For this review, take the finished solid that the model builds, in its own axes (mm). A direction names the side the tool comes from. Round coordinates to 2 decimals unless told otherwise and drop trailing zeros. Write each loop counter-clockwise with the first axis right and the second up, starting at its lowest first coordinate (ties: lowest second). Pieces come first, ordered by that corner, then holes. Notation, with made-up numbers: (47.5, -40) -> (94.5, -40) arc R31 cw to (94.5, -1) -> close; hole circle Ø8 at (14, -32.5). An arc over 180 degrees is marked (long way). Answer as CSV lines item,"result". Start each with the question number.
Item 1: Take a section at B-B on z = -17.75. Count the separate pieces of the cut face and the enclosed holes in it, then the cut area to 3 significant figures.
Item 2: Machinability: for faces 4 (the cylindrical face through (-28.95, -54.45, -25.09)), 5 (the cylindrical face through (5.325, 32.732, -13.727)), 6 (the flat face through (-7.605, -12.93, -4.93)), which of the approach directions +Z, -Z, +X, -X, +Y, -Y give a long, thin tool a straight path to every point of the face, cutting with its end or side? Answer none if there is none.
Item 3: Wall thickness on probe 1 along X at (y, z) = (-24, -4.5); probe 2 along X at (y, z) = (-38, -24.25); probe 3 along Y at (x, z) = (-32.5, -24.25): over which ranges is each line inside the solid? List them lowest first. Write a range as from..to.
Item 4: For pin 1 Ø8 at (y, z) = (14, -23) entering from -X; pin 2 Ø5.5 at (x, y) = (-65, 0) entering from -Z (3 decimals); pin 3 Ø5 at (y, z) = (-54.5, -9.5) entering from +X, all flat-tipped, find the tip position at first contact; note any pin that passes through.
Item 5: Mouldability with a two-part tool opening along X and no side actions: class faces 1 (the flat face through (15, 0, -5)), 2 (the flat face through (16, 1, 0)), 3 (the cylindrical face through (-9.764, 74.362, -13.348)) as +X half, -X half, draft (parallel to the pull), parting line (faces both ways), or undercut.
Item 6: Take a section at A-A on x = 65. Give the boundary of the cut face in (y, z) (3 decimals), then the cut area to 3 significant figures.
```python
from build123d import *

# Parameters (mm, degrees)
ESBO_O1_R                        = 75
RESSALTO_EXTRUS_O1_DEPTH         = 27.075013067
ESBO_O2_R                        = 8.8
CORTE_EXTRUS_O1_DEPTH            = 110.467147275
CORTE_EXTRUS_O2_DEPTH            = 10
REBAIXO_PARA_SHCS_M41_AT_2_COUNT = 2
REBAIXO_PARA_SHCS_M41_AT_2_PITCH = 65
REBAIXO_PARA_SHCS_M41_AT_3_COUNT = 2
REBAIXO_PARA_SHCS_M41_AT_3_PITCH = 112.583302492
REBAIXO_PARA_SHCS_M41_AT_4_COUNT = 2
REBAIXO_PARA_SHCS_M41_AT_4_PITCH = 130
REBAIXO_PARA_SHCS_M41_AT_5_COUNT = 2
REBAIXO_PARA_SHCS_M41_AT_5_PITCH = 65
REBAIXO_PARA_SHCS_M41_AT_6_COUNT = 2
REBAIXO_PARA_SHCS_M41_AT_6_PITCH = 112.583302492
CORTE_EXTRUS_O3_DEPTH            = 110.467147275
PADR_OCIRCULAR1_COUNT            = 5
ESBO_O9_R                        = 4


with BuildPart() as part:
    # Esboço1 → Ressalto-extrusão1 (new body)
    with BuildSketch(Plane.XY):
        Circle(ESBO_O1_R)
    extrude(amount=-RESSALTO_EXTRUS_O1_DEPTH)

    # Esboço2 → Corte-extrusão1 (cut, through all)
    with BuildSketch(Plane.XY):
        Circle(ESBO_O2_R)
    extrude(amount=-CORTE_EXTRUS_O1_DEPTH, mode=Mode.SUBTRACT)

    # Esboço3 → Corte-extrusão2 (cut)
    with BuildSketch(Plane.XY):
        Polygon((0, 17.320508076), (-15, 8.660254038), (-15, -8.660254038), (0, -17.320508076), (15, -8.660254038), (15, 8.660254038), align=None)
    extrude(amount=-CORTE_EXTRUS_O2_DEPTH, mode=Mode.SUBTRACT)

    # Esboço5 → Rebaixo para SHCS M41 (revolve, cut)
    with BuildSketch(Plane(origin=(65, 0, -27.075013067), x_dir=(0, 1, 0), z_dir=(1, 0, 0))):
        Polygon((0, 0), (0, 27.075013067), (2.4, 27.075013067), (2.4, 4), (4, 4), (4, 0.025), (4.025, 0), align=None)
    rebaixo_para_shcs_m41 = revolve(axis=Axis((65, 0, -33.425013067), (0, 0, 1)), mode=Mode.SUBTRACT)

    # Rebaixo para SHCS M41 at 2: Rebaixo para SHCS M41 ×2
    with Locations(*[Vector(-0.49999999999999795, 0.8660254037844399, 0) * (i * REBAIXO_PARA_SHCS_M41_AT_2_PITCH) for i in range(1, REBAIXO_PARA_SHCS_M41_AT_2_COUNT)]):
        add(rebaixo_para_shcs_m41, mode=Mode.SUBTRACT)

    # Rebaixo para SHCS M41 at 3: Rebaixo para SHCS M41 ×2
    with Locations(*[Vector(-0.866025403784438, 0.500000000000001, 0) * (i * REBAIXO_PARA_SHCS_M41_AT_3_PITCH) for i in range(1, REBAIXO_PARA_SHCS_M41_AT_3_COUNT)]):
        add(rebaixo_para_shcs_m41, mode=Mode.SUBTRACT)

    # Rebaixo para SHCS M41 at 4: Rebaixo para SHCS M41 ×2
    with Locations(*[(-i * REBAIXO_PARA_SHCS_M41_AT_4_PITCH, 0, 0) for i in range(1, REBAIXO_PARA_SHCS_M41_AT_4_COUNT)]):
        add(rebaixo_para_shcs_m41, mode=Mode.SUBTRACT)

    # Rebaixo para SHCS M41 at 5: Rebaixo para SHCS M41 ×2
    with Locations(*[Vector(-0.500000000000004, -0.8660254037844364, 0) * (i * REBAIXO_PARA_SHCS_M41_AT_5_PITCH) for i in range(1, REBAIXO_PARA_SHCS_M41_AT_5_COUNT)]):
        add(rebaixo_para_shcs_m41, mode=Mode.SUBTRACT)

    # Rebaixo para SHCS M41 at 6: Rebaixo para SHCS M41 ×2
    with Locations(*[Vector(-0.8660254037844416, -0.499999999999995, 0) * (i * REBAIXO_PARA_SHCS_M41_AT_6_PITCH) for i in range(1, REBAIXO_PARA_SHCS_M41_AT_6_COUNT)]):
        add(rebaixo_para_shcs_m41, mode=Mode.SUBTRACT)

    # Esboço6 → Corte-extrusão3 (cut, through all)
    with BuildSketch(Plane(origin=(0, 0, -27.075013067), x_dir=(-1, 0, 0), z_dir=(0, 0, -1))):
        with BuildLine():
            ThreePointArc((-1.875, 42.563377787), (-9.330127019, 41.160254038), (-6.817704321, 34.002362777))
            ThreePointArc((-6.817704321, 34.002362777), (-5.310250702, 32.70762802), (-4.942704321, 30.754767512))
            ThreePointArc((-4.942704321, 30.754767512), (0, 25), (4.942704321, 30.754767512))
            ThreePointArc((4.942704321, 30.754767512), (5.310250702, 32.70762802), (6.817704321, 34.002362777))
            ThreePointArc((6.817704321, 34.002362777), (9.330127019, 41.160254038), (1.875, 42.563377787))
            ThreePointArc((1.875, 42.563377787), (0, 41.905252036), (-1.875, 42.563377787))
        make_face()
    corte_extrus_o3 = extrude(amount=-CORTE_EXTRUS_O3_DEPTH, mode=Mode.SUBTRACT)

    # PadrãoCircular1: Corte-extrusão3 ×5 about axis
    padr_ocircular1_axis = Axis((0, 0, 0), (0, 0, 1))
    for i in range(1, PADR_OCIRCULAR1_COUNT):
        add(corte_extrus_o3.rotate(padr_ocircular1_axis, i * 360 / PADR_OCIRCULAR1_COUNT), mode=Mode.SUBTRACT)

    # Esboço9 → Corte-Revolução1 (revolve, cut)
    with BuildSketch(Plane(origin=(0, 0, 0), x_dir=(1, 0, 0), z_dir=(0, 1, 0)), mode=Mode.PRIVATE) as corte_revolu_o1_sk:
        with Locations((-53.5, 27.075013067)):
            Circle(ESBO_O9_R)
    revolve(corte_revolu_o1_sk.sketch.rotate(Axis((0, 0, -10), (0, 0, -1)), 180), axis=Axis((0, 0, -10), (0, 0, -1)), mode=Mode.SUBTRACT)


solid = part.part
```
Output values:
1,separate pieces,"1"
1,enclosed holes,"12"
1,area,"16,100 mm^2"
2,face 4,"-Z"
2,face 5,"+Z, -Z"
2,face 6,"+Z"
3,probe 1,"x = -71.06..-29.26, -12.64..12.64, 29.26..71.06"
3,probe 2,"x = -64.66..-41.58, -33.52..-21.95, -15.41..15.41, 21.95..33.52, 41.58..64.66"
3,probe 3,"y = -67.59..-60.29, -52.29..-46.01, -38.87..5.1, 20.9..38.87, 46.01..52.29, 60.29..67.59"
4,pin 1,"stops at x = -74.33"
4,pin 2,"stops at z = -23.075"
4,pin 3,"stops at x = 54.05"
5,face 1,"undercut"
5,face 2,"draft"
5,face 3,"parting line"
6,outline,"(-37.417, -27.075) -> (-4.025, -27.075) -> (-4, -27.05) -> (-4, -23.075) -> (-2.4, -23.075) -> (-2.4, 0) -> (-37.417, 0) -> close; (2.4, -23.075) -> (4, -23.075) -> (4, -27.05) -> (4.025, -27.075) -> (37.417, -27.075) -> (37.417, 0) -> (2.4, 0) -> close"
6,area,"1,880 mm^2"
